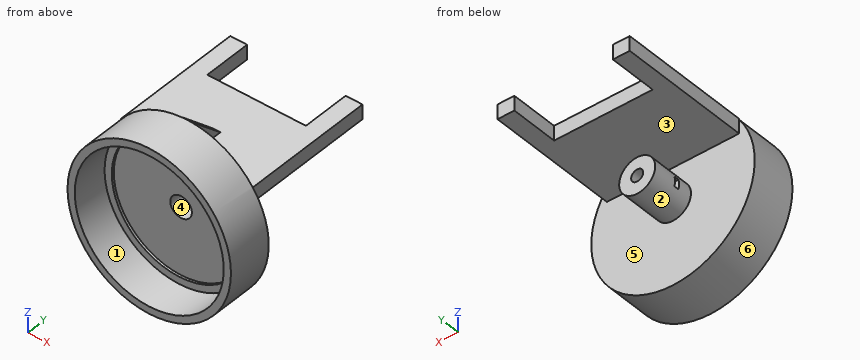
from build123d import *

# Parameters (mm, degrees)
SKETCH10_R              = 7.5
SKETCH10_R_2            = 4.5
BOSS_EXTRUDE2_DEPTH     = 8
CUT_EXTRUDE2_DEPTH      = 19
CUT_EXTRUDE2_DEPTH_BACK = 12
SKETCH11_W              = 4
SKETCH11_H              = 2
SKETCH13_R              = 7.5
SKETCH13_R_2            = 2.5
BOSS_EXTRUDE3_DEPTH     = 10
SKETCH15_W              = 55
SKETCH15_H              = 6.077899871
BOSS_EXTRUDE4_DEPTH     = 35
SKETCH16_W              = 7
SKETCH16_H              = 6.077899871
BOSS_EXTRUDE5_DEPTH     = 20


with BuildPart() as part:
    # Sketch2 → Revolve1 (revolve)
    with BuildSketch(Plane(origin=(0, 0, 0), x_dir=(0, 0, -1), z_dir=(1, 0, 0))):
        Polygon((31, 0), (31, -15), (34, -15), (34, 4), (31, 4), (4.5, 4), (4.5, 1), (28, 1), (28, 0), align=None)
    revolve(axis=Axis((0, 0, 0), (0, 1, 0)))

    # Sketch10 → Boss-Extrude2 (add)
    with BuildSketch(Plane(origin=(0, 4, 0), x_dir=(1, 0, 0), z_dir=(0, 1, 0))):
        with Locations(Location((0, 0, 0), (0, 0, 270))):
            Circle(SKETCH10_R)
        with Locations(Location((0, 0, 0), (0, 0, 90))):
            Circle(SKETCH10_R_2, mode=Mode.SUBTRACT)
    extrude(amount=BOSS_EXTRUDE2_DEPTH)

    # Sketch11 → Cut-Extrude2 (cut, two sides: drawn at the far end of the back side and taken through both)
    with BuildSketch(Plane(origin=(0, 0, 0), x_dir=(0, 0, -1), z_dir=(1, 0, 0)).offset(-CUT_EXTRUDE2_DEPTH_BACK)):
        with Locations((0, 11)):
            Rectangle(SKETCH11_W, SKETCH11_H)
    extrude(amount=CUT_EXTRUDE2_DEPTH + CUT_EXTRUDE2_DEPTH_BACK, mode=Mode.SUBTRACT)

    # Sketch13 → Boss-Extrude3 (add)
    with BuildSketch(Plane(origin=(0, 12, 0), x_dir=(1, 0, 0), z_dir=(0, 1, 0))):
        with Locations(Location((0, 0, 0), (0, 0, 270))):
            Circle(SKETCH13_R)
        with Locations(Location((0, 0, 0), (0, 0, 270))):
            Circle(SKETCH13_R_2, mode=Mode.SUBTRACT)
    extrude(amount=BOSS_EXTRUDE3_DEPTH)

    # Sketch15 → Boss-Extrude4 (add)
    with BuildSketch(Plane(origin=(0, 4, 0), x_dir=(1, 0, 0), z_dir=(0, 1, 0))):
        with Locations((0, -17.339890807)):
            Rectangle(SKETCH15_W, SKETCH15_H)
    extrude(amount=BOSS_EXTRUDE4_DEPTH)

    # Sketch16 → Boss-Extrude5 (add)
    with BuildSketch(Plane(origin=(0, 39, 0), x_dir=(1, 0, 0), z_dir=(0, 1, 0))):
        with Locations((24, -17.339890807)):
            Rectangle(SKETCH16_W, SKETCH16_H)
        with Locations((-24, -17.339890807)):
            Rectangle(SKETCH16_W, SKETCH16_H)
    extrude(amount=BOSS_EXTRUDE5_DEPTH)

    # Loft1: read off the stored shape, not the designer's step
    # Loft1: loft between two sections, ruled curve by curve
    loft1_from = [
        Edge.make_bspline([(-2.096925142, 4, 24), (-2.096925142, 4, 25.666666667), (-2.096925142, 4, 27.333333333), (-2.096925142, 4, 30.666666667), (-2.096925142, 4, 32.333333333), (-2.096925142, 4, 34)], [0, 0, 0, 0, 0.5, 0.5, 1, 1, 1, 1], 3),
        Edge.make_bspline([(2.096925142, 4, 34), (2.096925142, 4, 32.333333333), (2.096925142, 4, 30.666666667), (2.096925142, 4, 27.333333333), (2.096925142, 4, 25.666666667), (2.096925142, 4, 24)], [0, 0, 0, 0, 0.5, 0.5, 1, 1, 1, 1], 3),
        Edge.make_line((-2.096925142, 4, 24), (2.096925142, 4, 24)),
        Edge.make_line((2.096925142, 4, 34), (-2.096925142, 4, 34)),
    ]
    loft1_to = [
        Edge.make_bspline([(-1.5, 14, 20.378840742), (-1.5, 14.833333333, 20.378840742), (-1.5, 15.666666667, 20.378840742), (-1.5, 17.333333333, 20.378840742), (-1.5, 18.166666667, 20.378840742), (-1.5, 19, 20.378840742)], [0, 0, 0, 0, 0.5, 0.5, 1, 1, 1, 1], 3),
        Edge.make_bspline([(1.5, 19, 20.378840742), (1.5, 18.166666667, 20.378840742), (1.5, 17.333333333, 20.378840742), (1.5, 15.666666667, 20.378840742), (1.5, 14.833333333, 20.378840742), (1.5, 14, 20.378840742)], [0, 0, 0, 0, 0.5, 0.5, 1, 1, 1, 1], 3),
        Edge.make_line((-1.5, 14, 20.378840742), (1.5, 14, 20.378840742)),
        Edge.make_line((1.5, 19, 20.378840742), (-1.5, 19, 20.378840742)),
    ]
    loft1 = Solid(Shell([*[Face.make_surface_from_curves(loft1_from[k], loft1_to[k]) for k in range(4)], Face(Wire(loft1_from)), Face(Wire(loft1_to))]))
    add(loft1)


solid = part.part
Input: part model. Units: mm. Frame: model coordinates. Face numbers are marked on the shaded views. A direction names the side the tool comes from. Round coordinates to 2 decimals unless told otherwise and drop trailing zeros. Order: outer loops, then holes, each group sorted by start corner. A loop starts at its lowest first (then second) coordinate and runs counter-clockwise, first axis right, second up.
1. Cut plane B-B, the plane z = 0. Output: boundary loops of the cut face in (x, y), then the cut area to 3 significant figures.
The answers:
outline: (-34, -15) - (-31, -15) - (-31, 0) - (-28, 0) - (-28, 1) - (-4.5, 1) - (-4.5, 10) - (-7.5, 10) - (-7.5, 4) - (-34, 4) - close; (-7.5, 12) - (-2.5, 12) - (-2.5, 22) - (-7.5, 22) - close; (2.5, 12) - (7.5, 12) - (7.5, 22) - (2.5, 22) - close; (4.5, 1) - (28, 1) - (28, 0) - (31, 0) - (31, -15) - (34, -15) - (34, 4) - (7.5, 4) - (7.5, 10) - (4.5, 10) - close
area: 415 mm2
2. Mould query, pull axis X, two halves, no side actions, for the marked faces 4, 5 and 6. Classes: released by +X, released by -X, zero draft, split by the parting line, or undercut.
The answers:
face 4: undercut
face 5: zero draft
face 6: split by the parting line
3. Pin query (flat end, axial travel): P1, Ø1.5, axis at y = 4.5, z = 1, coming from the -X side; P2, Ø15, axis at x = -10.5, z = 29, coming from the +Y side; P3, Ø7, axis at x = 1, z = 1, coming from the -Y side; P4, Ø3, axis at x = 0, z = 0, coming from the -Y side. Return the tip coordinate at first contact, or that it passes through.
The answers:
P1: stops at x = -34
P2: stops at y = 4
P3: stops at y = 1
P4: passes through
4. Cut plane A-A, the plane y = 54. Output: boundary loops of the cut face in (x, z).
The answers:
outline: (-27.5, 14.3) - (-20.5, 14.3) - (-20.5, 20.38) - (-27.5, 20.38) - close; (20.5, 14.3) - (27.5, 14.3) - (27.5, 20.38) - (20.5, 20.38) - close
5. Material intervals for line 1 (X direction, y = 15.5, z = 0); line 2 (Y direction, x = 2, z = 2); line 3 (Z direction, x = -13.5, y = 38), sorted ascending.
The answers:
line 1: x = -7.5 to -2.5, 2.5 to 7.5
line 2: y = 12 to 22
line 3: z = 14.3 to 20.38
6. Cut plane D-D, the plane z = 18.5. Output: boundary loops of the cut face in (x, y), then the cut area to 3 significant figures.
The answers:
outline: (-28.53, -15) - (-24.87, -15) - (-24.87, 0) - (-21.02, 0) - (-21.02, 1) - (21.02, 1) - (21.02, 0) - (24.87, 0) - (24.87, -15) - (28.53, -15) - (28.53, 4) - (27.5, 4) - (27.5, 59) - (20.5, 59) - (20.5, 39) - (-20.5, 39) - (-20.5, 59) - (-27.5, 59) - (-27.5, 4) - (-28.53, 4) - close
area: 2,500 mm2
7. Cut plane C-C, the plane x = -14. Output: boundary loops of the cut face in (y, z), then the cut area to 3 significant figures.
The answers:
outline: (-15, -30.98) - (4, -30.98) - (4, 14.3) - (39, 14.3) - (39, 20.38) - (4, 20.38) - (4, 30.98) - (-15, 30.98) - (-15, 27.66) - (0, 27.66) - (0, 24.25) - (1, 24.25) - (1, -24.25) - (0, -24.25) - (0, -27.66) - (-15, -27.66) - close
area: 512 mm2
8. Set-up query: the marked faces 1, 2 and 3. Return all of +Z, -Z, +X, -X, +Y, -Y with unobstructed straight access to the full face (end or side cutting, diameter ignored); none if empty.
The answers:
face 1: -Y
face 2: +Y
face 3: +X, -X, +Y
